CAD build for the part. Positions are in the model's coordinates, mm. Face numbers are marked on the shaded views. A direction names the side the tool comes from. Round coordinates to 2 decimals unless told otherwise and drop trailing zeros. Order: outer loops, then holes, each group sorted by start corner. A loop starts at its lowest first (then second) coordinate and runs counter-clockwise, first axis right, second up. Notation, with made-up numbers: M 24.5,-26 L 36.5,-26 A21 cw 36.5,-4 Z; hole C 48.25,45 d10. An arc over 180 degrees is marked long. Answer as a JSON object with one key per item and string values.
```python
from build123d import *

# Parameters (mm, degrees)
SKETCH2_W             = 40
SKETCH2_H             = 32.5
BOSS_EXTRUDE1_DEPTH   = 25
SKETCH3_W             = 40
SKETCH3_H             = 5
BOSS_EXTRUDE2_DEPTH   = 25
SKETCH1_R             = 14
CUT_EXTRUDE1_DEPTH    = 9
CHAMFER1_SIZE         = 1
M4_TAPPED_HOLE2_D     = 3.3
M4_TAPPED_HOLE2_DEPTH = 10
M4_TAPPED_HOLE2_TIP   = 0.991420021
CHAMFER2_SIZE         = 5
M4_TAPPED_HOLE3_D     = 3.3
M4_TAPPED_HOLE3_DEPTH = 12.1
M4_TAPPED_HOLE3_TIP   = 0.991420021


with BuildPart() as part:
    # Sketch2 → Boss-Extrude1 (new body)
    with BuildSketch(Plane(origin=(0, 0, 0), x_dir=(1, 0, 0), z_dir=(0, 1, 0))):
        with Locations((0, 3.75)):
            Rectangle(SKETCH2_W, SKETCH2_H)
    extrude(amount=BOSS_EXTRUDE1_DEPTH)

    # Sketch3 → Boss-Extrude2 (add)
    with BuildSketch(Plane.XZ):
        with Locations((0, 15)):
            Rectangle(SKETCH3_W, SKETCH3_H)
    extrude(amount=-BOSS_EXTRUDE2_DEPTH)

    # Sketch1 → Cut-Extrude1 (cut)
    with BuildSketch(Plane(origin=(0, 0, 0), x_dir=(1, 0, 0), z_dir=(0, 1, 0))):
        with Locations(Location((0, 0, 0), (0, 0, 270))):
            Circle(SKETCH1_R)
    extrude(amount=CUT_EXTRUDE1_DEPTH, mode=Mode.SUBTRACT)

    # Chamfer1
    chamfer1_edges = [part.edges().sort_by_distance(p)[0] for p in [
        (0, 0, -14),
    ]]
    chamfer(chamfer1_edges, length=CHAMFER1_SIZE)

    # M4 Tapped Hole2
    with Locations(Plane(origin=(0, 0, -20), x_dir=(-1, 0, 0), z_dir=(0, 0, -1))):
        with Locations((0, 17)):
            Hole(M4_TAPPED_HOLE2_D / 2, depth=M4_TAPPED_HOLE2_DEPTH)
            with Locations((0, 0, -(M4_TAPPED_HOLE2_DEPTH + M4_TAPPED_HOLE2_TIP / 2))):  # 118° drill point
                Cone(0, M4_TAPPED_HOLE2_D / 2, M4_TAPPED_HOLE2_TIP, mode=Mode.SUBTRACT)

    # Chamfer2
    chamfer2_edges = [part.edges().sort_by_distance(p)[0] for p in [
        (20, 12.5, 17.5),
        (-20, 12.5, 17.5),
    ]]
    chamfer(chamfer2_edges, length=CHAMFER2_SIZE)

    # M4 Tapped Hole3
    with Locations(Plane(origin=(0, 25, 0), x_dir=(1, 0, 0), z_dir=(0, 1, 0))):
        with Locations((-16, 15), (-16, -7.5), (16, -7.5), (16, 15)):
            Hole(M4_TAPPED_HOLE3_D / 2, depth=M4_TAPPED_HOLE3_DEPTH)
            with Locations((0, 0, -(M4_TAPPED_HOLE3_DEPTH + M4_TAPPED_HOLE3_TIP / 2))):  # 118° drill point
                Cone(0, M4_TAPPED_HOLE3_D / 2, M4_TAPPED_HOLE3_TIP, mode=Mode.SUBTRACT)


solid = part.part
```
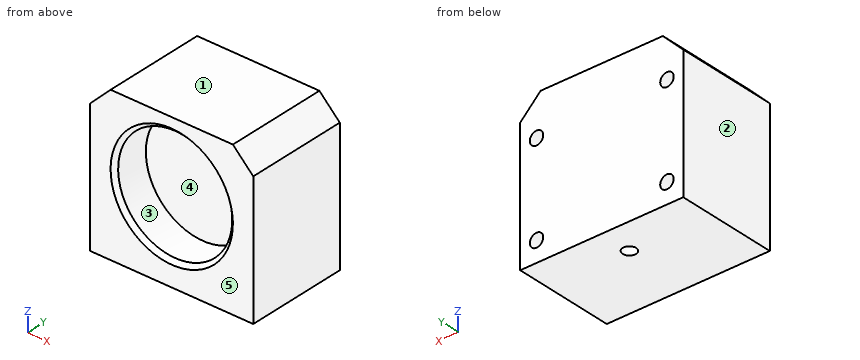
Item 1: Saw through at A-A on y = 4. List the corners of the cut face in (x, z).
Worked answers:
{"outline": "M -20,-20 L 20,-20 L 20,12.5 L 15,17.5 L -15,17.5 L -20,12.5 Z; hole C 0,0 d28"}
Item 2: Wall check: line 1 along X through (y, z) = (18, 7.5); line 2 along Z through (x, y) = (-14.5, 23); line 3 along Z through (x, y) = (-16, 16.5). Give the ranges that are in metal, low to high. Write a range as [from, to].
Worked answers:
{"line 1": "x = [-20, -17.65], [-14.35, 14.35], [17.65, 20]", "line 2": "z = [-20, -15.69], [-14.31, 6.81], [8.19, 17.5]", "line 3": "z = [-20, -16.65], [-13.35, 5.85], [9.15, 16.5]"}
Item 3: Saw through at D-D on y = 17.5. State how many separate pieces and enclosed holes the cut face has, and give its area (3 significant figures).
Worked answers:
{"separate pieces": "1", "enclosed holes": "4", "area": "1,410 mm2"}
Item 4: 3-axis set-ups, long thin cutter, end or side, ignore diameter. For the marked faces 4 and 5: which of +Z, -Z, +X, -X, +Y, -Y reach the whole face in a straight line?
Worked answers:
{"face 4": "-Y", "face 5": "+Z, -Z, +X, -X, -Y"}
Item 5: Drop flat-ended pins along their axis: pin 1 Ø3 at (x, z) = (-5, -6) entering from -Y; pin 2 Ø3 at (x, z) = (-16, -15) entering from +Y. Give the stop position or say it passes through.
Worked answers:
{"pin 1": "stops at y = 9", "pin 2": "stops at y = 12.81"}
Item 6: Saw through at B-B on z = 0. List the corners of the cut face in (x, y).
Worked answers:
{"outline": "M -20,0 L -15,0 L -14,1 L -14,9 L 14,9 L 14,1 L 15,0 L 20,0 L 20,25 L -20,25 Z"}
Item 7: Two-plate mould, pull along X, no slides. Class the marked faces 1, 2 and 3: released by +X, released by -X, zero draft, split by the parting line, or undercut.
Worked answers:
{"face 1": "zero draft", "face 2": "released by -X", "face 3": "undercut"}
Item 8: Saw through at C-C on y = 14.25. List the corners of the cut face in (x, z).
Worked answers:
{"outline": "M -20,-20 L 20,-20 L 20,12.5 L 15,17.5 L -15,17.5 L -20,12.5 Z; hole C -16,-15 d3.3; hole C -16,7.5 d3.3; hole C 16,-15 d3.3; hole C 16,7.5 d3.3"}
